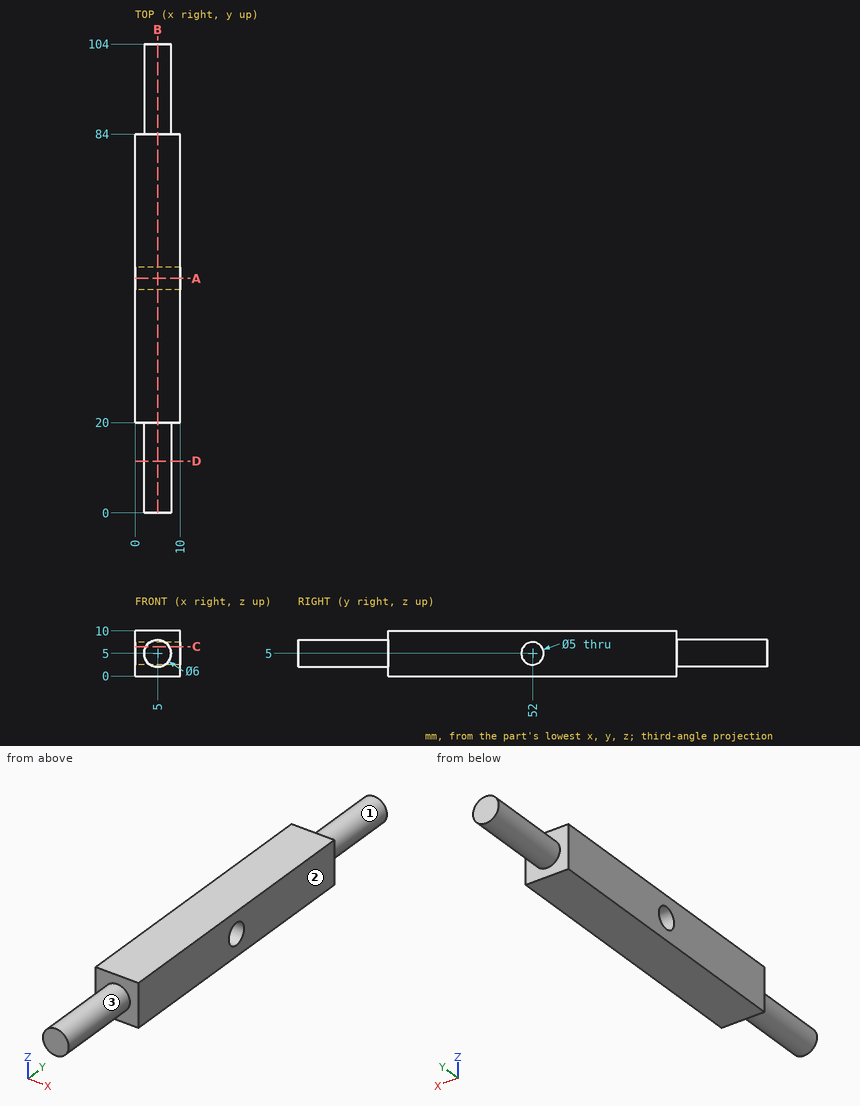
The figure shows three views and two pictorial views of one solid part (mm, origin at its lowest corner). Answer the questions. A direction names the side the tool comes from. Coordinates: 2 decimals unless noted, no trailing zeros. Order: outer loops, then holes, each group sorted by start corner. A loop starts at its lowest first (then second) coordinate and runs counter-clockwise, first axis right, second up.
Q1. A cutting plane is placed at D-D, the plane y = 11.5. Write down the section's boundary in (x, z), and give its area (3 significant figures).
Q2. A cutting plane is placed at C-C, the plane z = 6.5. Write down the section's boundary in (x, y), and give its area (3 significant figures).
Q3. A cutting plane is placed at B-B, the plane x = 5. Write down the section's boundary in (y, z), and give its area (3 significant figures).
Q4. Which of the six approach directions +Z, -Z, +X, -X, +Y, -Y give full straight-line access (tool end or side, diameter ignored) to the marked faces 1, 2 and 3?
Q5. A cutting plane is placed at A-A, the plane y = 52. Write down the section's boundary in (x, z).
Q6. Consider line 1 (Z direction, x = 6, y = 52); line 2 (Y direction, x = 9, z = 6.5); line 3 (Y direction, x = 4, z = 8.5). Determine where each line is inside the solid, lowest interval first.
Q7. Given P1, Ø4, axis at x = 2.5, y = 14, coming from the -Z side; P2, Ø2, axis at x = 2, y = 17.5, coming from the +Z side; P3, Ø4, axis at y = 52, z = 5, coming from the -X side; P4, Ø2, axis at x = 2, z = 9, coming from the -Y side, each flat-ended and moving along its own axis, determine where each tip first touches the part or whether it passes through.
Answers follow:
1. outline: circle Ø6 at (5, 5)
1. area: 28.3 mm2
2. outline: (0, 20) - (2.4, 20) - (2.4, 0) - (7.6, 0) - (7.6, 20) - (10, 20) - (10, 50) - (0, 50) - close; (0, 54) - (10, 54) - (10, 84) - (7.6, 84) - (7.6, 104) - (2.4, 104) - (2.4, 84) - (0, 84) - close
2. area: 808 mm2
3. outline: (0, 2) - (20, 2) - (20, 0) - (84, 0) - (84, 2) - (104, 2) - (104, 8) - (84, 8) - (84, 10) - (20, 10) - (20, 8) - (0, 8) - close; hole circle Ø5 at (52, 5)
3. area: 860 mm2
4. face 1: +Y
4. face 2: +Z, -Z, +X, +Y, -Y
4. face 3: -Y
5. outline: (0, 0) - (10, 0) - (10, 2.5) - (0, 2.5) - close; (0, 7.5) - (10, 7.5) - (10, 10) - (0, 10) - close
6. line 1: z = 0 to 2.5, 7.5 to 10
6. line 2: y = 20 to 50, 54 to 84
6. line 3: y = 20 to 84
7. P1: stops at z = 2.04
7. P2: stops at z = 7.24
7. P3: passes through
7. P4: stops at y = 20
